from build123d import *

# Parameters (mm, degrees)
BOSS_EXTRUDE1_DEPTH = 3
SKETCH2_W           = 138.4
SKETCH2_H           = 3
CUT_EXTRUDE1_DEPTH  = 4
SKETCH3_W           = 19.771429
SKETCH3_H           = 3
BOSS_EXTRUDE2_DEPTH = 3


with BuildPart() as part:
    # Sketch1 → Boss-Extrude1 (new body)
    with BuildSketch(Plane(origin=(0, 0, 0), x_dir=(1, 0, 0), z_dir=(0, 1, 0))):
        Polygon((0, 0), (28.88, 0), (28.88, -3), (57.76, -3), (57.76, 0), (86.64, 0), (86.64, -3), (115.52, -3), (115.52, 0), (144.4, 0), (144.4, 22.85), (141.4, 22.85), (141.4, 45.68), (144.4, 45.68), (144.4, 68.51), (141.4, 68.51), (141.4, 91.34), (144.4, 91.34), (144.4, 114.17), (141.4, 114.17), (141.4, 137), (3, 137), (3, 114.17), (0, 114.17), (0, 91.34), (3, 91.34), (3, 68.51), (0, 68.51), (0, 45.68), (3, 45.68), (3, 22.85), (0, 22.85), align=None)
    extrude(amount=BOSS_EXTRUDE1_DEPTH)

    # Sketch2 → Cut-Extrude1 (cut, through all)
    with BuildSketch(Plane.XZ):
        with Locations((72.2, -135.5)):
            Rectangle(SKETCH2_W, SKETCH2_H)
    extrude(amount=-CUT_EXTRUDE1_DEPTH, mode=Mode.SUBTRACT)

    # Sketch3 → Boss-Extrude2 (add)
    with BuildSketch(Plane.XZ):
        with Locations((32.657143071, -135.5)):
            Rectangle(SKETCH3_W, SKETCH3_H)
        with Locations((72.200001071, -135.5)):
            Rectangle(SKETCH3_W, SKETCH3_H)
        with Locations((111.742859071, -135.5)):
            Rectangle(SKETCH3_W, SKETCH3_H)
    extrude(amount=-BOSS_EXTRUDE2_DEPTH)


solid = part.part
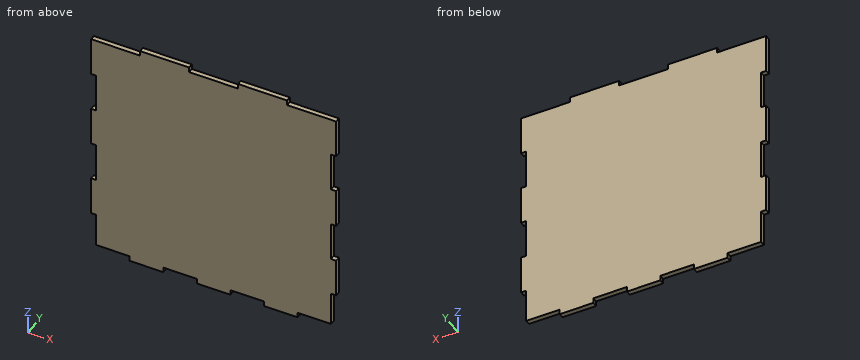
Here's how the part is built. I have some questions about the finished solid (model axes, mm). Coordinates: 2 decimals unless noted, no trailing zeros. Write each loop counter-clockwise with the first axis right and the second up, starting at its lowest first coordinate (ties: lowest second). Pieces come first, ordered by that corner, then holes. Notation, with made-up numbers: (54, 33.25) - (87, 33.25) arc R14 cw to (87, 58.25) - close; hole circle Ø9 at (-21.5, 3). An arc over 180 degrees is marked (long way). Use one line per item in the form item = value.
1) Suppose I cut it at A-A, the plane x = 21. Write out the boundary of the cut face in (y, z), plus the area to 3 significant figures.
Solved:
outline = (0, -134) - (3, -134) - (3, 0) - (0, 0) - close
area = 402 mm2
2) I need wall thicknesses on line 1 (X direction, y = 2.6, z = -120); line 2 (Z direction, x = 52, y = 2.2); line 3 (Z direction, x = 72, y = 2.5). Which ranges of each line are inside material? Lowest first, please.
Solved:
line_1 = 3 to 141.4
line_2 = -134 to 3
line_3 = -137 to 0
3) I'm going to push flat-ended pins straight in: P1, Ø0.9, axis at y = 1.5, z = 1, coming from the +X side; P2, Ø1.5, axis at y = 1, z = -135.5, coming from the +X side; P3, Ø0.9, axis at x = 143.5, y = 2, coming from the -Z side. Where does each tip first touch, or does it pass through?
Solved:
P1 = 115.52
P2 = 121.63
P3 = -114.17
4) Suppose I cut it at B-B, the plane z = -31. Write out the boundary of the cut face in (x, y).
Solved:
outline = (3, 0) - (141.4, 0) - (141.4, 3) - (3, 3) - close
